Study the drawing (mm; zero at the part's minimum x, y, z) and answer. Give positions to 0.01 mm unless a question says otherwise; leave off trailing zeros. Write each loop counter-clockwise with the first axis right and the second up, starting at its lowest first coordinate (ties: lowest second). Pieces come first, ordered by that corner, then holes.
1) Find section A-A (y = 16). Determine the outline of the cut face in (x, z) (3 decimals), plus the area to 3 significant figures.
2) Given pin 1 Ø6 at (x, z) = (76, 52) entering from -Y; pin 2 Ø4 at (x, y) = (87, 13) entering from +Z (3 decimals); pin 3 Ø2.5 at (x, y) = (88, 13) entering from -Z (3 decimals), each flat-ended and moving along its own axis, determine where each tip first touches the part or whether it passes through.
3) Find section C-C (x = 62). Determine the outline of the cut face in (y, z), plus the area to 3 significant figures.
4) Determine the mould class of the marked faces 1, 2, 3 and 4 for opening direction X: pulls with the +X half, pulls with the -X half, needs draft (parallel to the pull), parting line crosses it, or undercut.
5) A straight line is drawn through the part: probe 1 along Y at (x, z) = (30, 28). Find the intervals that lie inside material, in ascending order.
6) Find section B-B (z = 34.5). Determine the outline of the cut face in (x, y), plus the area to 3 significant figures.
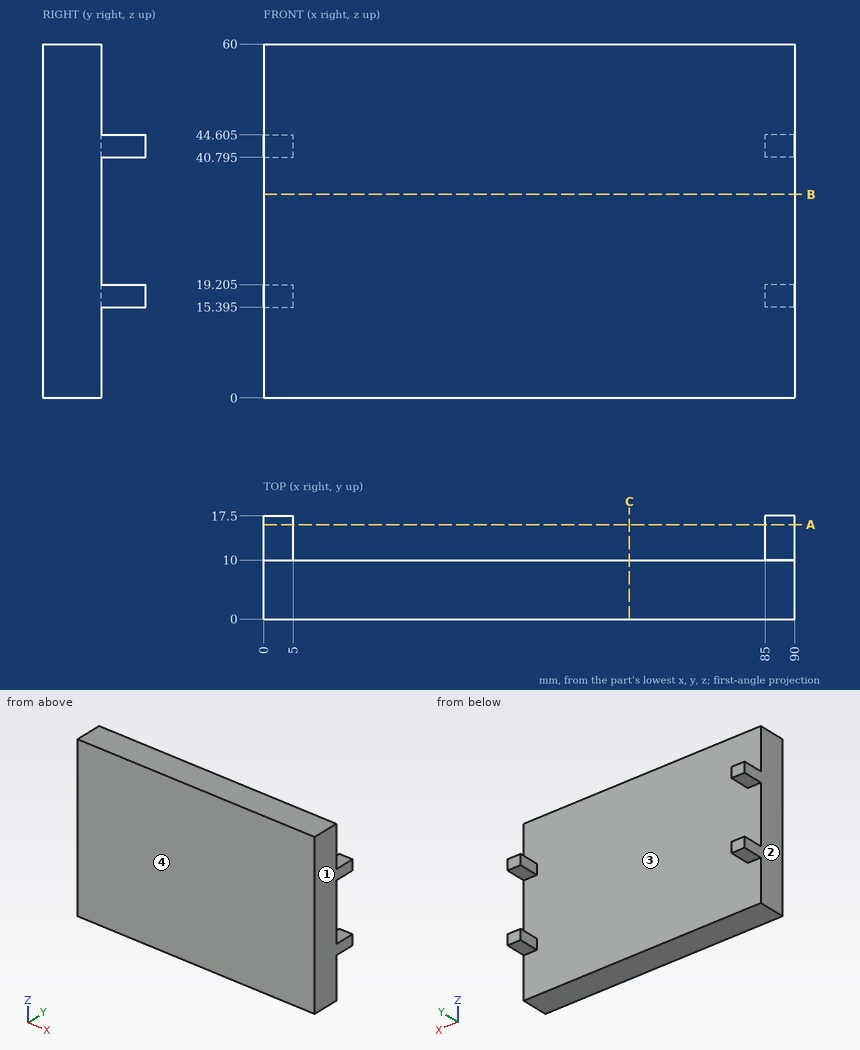
Results:
1. outline: (0, 15.395) - (5, 15.395) - (5, 19.205) - (0, 19.205) - close; (0, 40.795) - (5, 40.795) - (5, 44.605) - (0, 44.605) - close; (85, 15.395) - (90, 15.395) - (90, 19.205) - (85, 19.205) - close; (85, 40.795) - (90, 40.795) - (90, 44.605) - (85, 44.605) - close
1. area: 76.2 mm2
2. pin 1: stops at y = 0
2. pin 2: stops at z = 44.605
2. pin 3: stops at z = 15.395
3. outline: (0, 0) - (10, 0) - (10, 60) - (0, 60) - close
3. area: 600 mm2
4. face 1: pulls with the +X half
4. face 2: pulls with the -X half
4. face 3: undercut
4. face 4: needs draft
5. probe 1: y = 0 to 10
6. outline: (0, 0) - (90, 0) - (90, 10) - (0, 10) - close
6. area: 900 mm2
